Can you work these out from the model? Positions are in its coordinate system, mm. A direction names the side the tool comes from. Give positions to 0.01 mm unless a question says otherwise; leave off trailing zeros. Order: outer loops, then holes, each group sorted by start corner. A loop starts at its lowest first (then second) coordinate and runs counter-clockwise, first axis right, second up. Notation, with made-up numbers: M -36.75,-7 L 3.25,-7 A29 ccw 3.25,28 Z; hole C 40,67.25 d9. An arc over 180 degrees is marked long. Use a Markdown table: item, result. Add a question column.
from build123d import *

# Parameters (mm, degrees)
F0_R     = 1
F1_DEPTH = 5
F2_DEPTH = 5
F3_COUNT = 11


with BuildPart() as f1:
    # F0 (on Top) → F1 (new body)
    with BuildSketch(Plane.XY):
        with BuildLine():
            ThreePointArc((4, 0), (3.1085838458, 2.5172815642), (0.8316467633, 3.9125904029))
            ThreePointArc((0.8316467633, 3.9125904029), (0.5221047689, 3.9657794455), (0.209343825, 3.994518139))
            ThreePointArc((0.209343825, 3.994518139), (-2.901497484, -2.7534183028), (4, 0))
        make_face()
        Circle(F0_R, mode=Mode.SUBTRACT)
    extrude(amount=F1_DEPTH)

    # F0 (on Top) → F2 (join)
    with BuildSketch(Plane.XY):
        with BuildLine():
            Line((1.1448017618, 5.8897732491), (1.4250798414, 9.8979365246))
            ThreePointArc((1.4250798414, 9.8979365246), (1.3052619222, 9.9144486137), (1.1852530565, 9.9295103199))
            Line((1.1852530565, 9.9295103199), (0.4185919005, 5.9853805911))
            Line((0.4185919005, 5.9853805911), (0.209343825, 3.994518139))
            ThreePointArc((0.209343825, 3.994518139), (0.5221047689, 3.9657794455), (0.8316467633, 3.9125904029))
            Line((0.8316467633, 3.9125904029), (1.1448017618, 5.8897732491))
        make_face()
    extrude(amount=F2_DEPTH)

    # F3: F1 ×11 about axis
    f3_axis = Axis((0, 0, 0), (0, 0, -1))


with BuildPart() as f1_1:
    add(f1.part)
    for i in range(1, F3_COUNT):
        add(f1.part.rotate(f3_axis, i * 360 / F3_COUNT))


solid = f1_1.part
1. We'd pull the mould along X, two halves only. Please class faces 6 (the face through (-3.02, -7.43, 2.46)), 7 (the face through (7.69, 2.1, 2.46)), 8 (the face through (4.996, 6.281, 2.465)), 9 (the face through (-4.421, 2.366, 2.465)): +X half, -X half, draft (parallel to the pull), parting line (faces both ways), or undercut.
2. If we section it at B-B, the plane y = -7: List the corners of the cut face in (x, z) for me, then the cut area to 3 significant figures.
3. If we section it at D-D, the plane x = 2: List the corners of the cut face in (y, z) for me, then the cut area to 3 significant figures.
4. Will these pins go through, and if not, where does the flat tip stop? pin 1 (1.5 mm diameter, centred on x = -6, z = 2.5, fed in from +Y); pin 2 (1.5 mm diameter, centred on x = -3.5, z = 2, fed in from -Y).
5. If we section it at C-C, the plane y = 8.25: List the corners of the cut face in (x, z) for me, then the cut area to 3 significant figures.
6. On a 3-axis mill with a long thin cutter (end or side, diameter ignored), from which of +Z, -Z, +X, -X, +Y, -Y can I reach the whole of each face in a straight line? I mean faces 1 (the face through (-6.928, 4.051, 2.465)), 2 (the face through (5.33, 5.92, 2.46)), 3 (the face through (2.97, 4.04, 2.46)), 4 (the face through (3.05, -3.95, 2.46)), 5 (the face through (1.475, -7.889, 2.465)). Say none if no direction works.
7. I need wall thicknesses on L1, parallel to X at y = 7.25, z = 1.9; L2, parallel to Y at x = 5, z = 1.9 (3 decimals); L3, parallel to Y at x = 0, z = 1.4. Which ranges of each line are inside material? Lowest first, please. Write a range as [from, to].
8. If we section it at A-A, the plane x = -7: List the corners of the cut face in (y, z) for me, then the cut area to 3 significant figures.
Geometry results:
| question | item | result |
|---|---|---|
| 1 | face 6 | undercut |
| 1 | face 7 | +X half |
| 1 | face 8 | undercut |
| 1 | face 9 | -X half |
| 2 | outline | M -3.38,0 L -2.8,0 L -2.8,5 L -3.38,5 Z; M 0.79,0 L 1.39,0 L 1.39,5 L 0.79,5 Z; M 5.99,0 L 6.42,0 L 6.42,5 L 5.99,5 Z |
| 2 | area | 8.07 mm^2 |
| 3 | outline | M -3.46,0 L 3.46,0 L 3.46,5 L -3.46,5 Z |
| 3 | area | 34.6 mm^2 |
| 4 | pin 1 | stops at y = 4.5 |
| 4 | pin 2 | stops at y = -9.19 |
| 5 | outline | M -4.07,0 L -3.69,0 L -3.69,5 L -4.07,5 Z; M 0.86,0 L 1.31,0 L 1.31,5 L 0.86,5 Z |
| 5 | area | 4.19 mm^2 |
| 6 | face 1 | +Z, -Z, -X |
| 6 | face 2 | +Z, -Z, +X |
| 6 | face 3 | +Z, -Z, +Y |
| 6 | face 4 | +Z, -Z, -Y |
| 6 | face 5 | +Z, -Z |
| 7 | L1 | x = [-3.68, -3.14], [0.66, 1.24], [5.92, 6.32] |
| 7 | L2 | y = [-6.017, -5.194], [-1.765, -1.048], [1.174, 1.898], [5.479, 6.285] |
| 7 | L3 | y = [-4, -1], [1, 4] |
| 8 | outline | M -4.87,0 L -4.34,0 L -4.34,5 L -4.87,5 Z; M -0.39,0 L 0.22,0 L 0.22,5 L -0.39,5 Z; M 4.1,0 L 4.64,0 L 4.64,5 L 4.1,5 Z |
| 8 | area | 8.37 mm^2 |
